Check sheet for the drawn part. Datum: minimum x, y, z corner. Units: mm. Coordinates: 2 decimals unless noted, no trailing zeros. Order: outer loops, then holes, each group sorted by start corner. A loop starts at its lowest first (then second) coordinate and runs counter-clockwise, first axis right, second up.
1. Thickness scan on line 1 (Z direction, x = 4.25, y = 132); line 2 (Y direction, x = 5.5, z = 134); line 3 (Y direction, x = 0.7, z = 163.5). Record the ranges inside material, lowest first.
2. Gauge pin test, flat end, axial feed: pin 1 Ø3 at (y, z) = (209.5, 143) entering from -X. Record the tip position at first contact, or that the pin passes through.
3. Cross-section at C-C (x = 4.55). Enter the section's corners in (y, z), then the cut area to 3 significant figures.
4. Cross-section at B-B (z = 147). Enter the section's corners in (x, y).
5. Cross-section at A-A (y = 132). Enter the section's corners in (x, z), then the cut area to 3 significant figures.
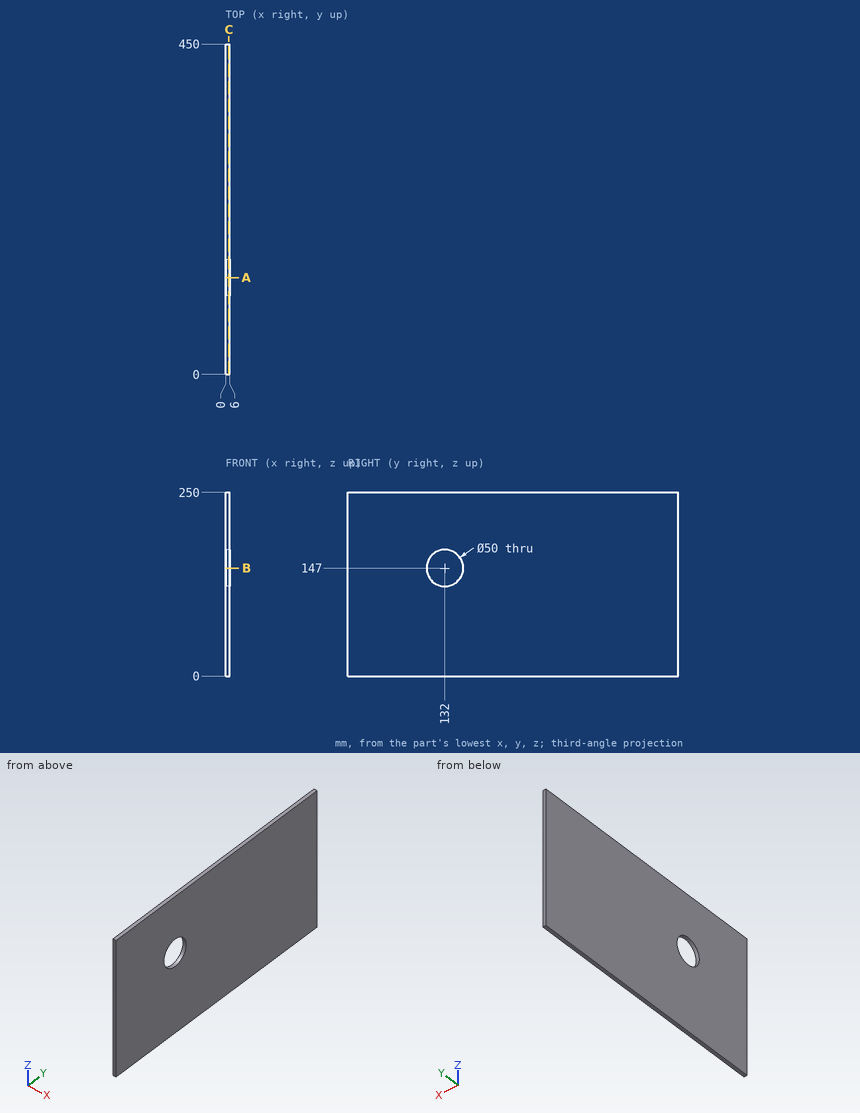
Data:
1. line 1: z = 0 to 122, 172 to 250
1. line 2: y = 0 to 110.65, 153.35 to 450
1. line 3: y = 0 to 113.22, 150.78 to 450
2. pin 1: stops at x = 0
3. outline: (0, 0) - (450, 0) - (450, 250) - (0, 250) - close; hole circle Ø50 at (132, 147)
3. area: 111,000 mm2
4. outline: (0, 0) - (6, 0) - (6, 107) - (0, 107) - close; (0, 157) - (6, 157) - (6, 450) - (0, 450) - close
5. outline: (0, 0) - (6, 0) - (6, 122) - (0, 122) - close; (0, 172) - (6, 172) - (6, 250) - (0, 250) - close
5. area: 1,200 mm2
